Check sheet for the drawn part. Datum: minimum x, y, z corner. Units: mm. A direction names the side the tool comes from. Coordinates: 2 decimals unless noted, no trailing zeros. Loops run counter-clockwise (first coordinate to the right, second up) from the corner with the lowest first, then second, coordinate; pieces in that order, holes last.
Q1. Sectioned sample at D-D (x = 23.5). Enter the section's corners in (y, z).
Q2. Mould release check, pull along Z, two halves, no side actions. Record for the marked faces 1, 2 and 3: +Z half, -Z half, draft (parallel to the pull), parting line (faces both ways), or undercut.
Q3. Sectioned sample at C-C (z = 13.25). Enter the section's corners in (x, y), then the cut area to 3 significant figures.
Q4. Sectioned sample at B-B (y = 2.25). Count the separate pieces of the cut face and the enclosed holes in it, then the cut area to 3 significant figures.
Q5. Material ranges on probe 1 along X at (y, z) = (2.9, 13.25); probe 2 along X at (y, z) = (8.5, 13.25); probe 3 along Z at (x, y) = (42, 2.05), recorded low to high.
Q6. Access from +Z, -Z, +X, -X, +Y, -Y to the whole of each face (thin tool, end or side, straight path). Record for the marked faces 4, 5 and 6.
Q7. Go/stop test with flat-tipped pins: P1, Ø1.2, axis at x = 41.5, y = 2.5, coming from the +Z side; P2, Ø5, axis at x = 23.5, z = 13.25, coming from the +Y side; P3, Ø3.5, axis at x = 42, z = 12, coming from the +Y side; P4, Ø1.2, axis at x = 5.5, y = 2, coming from the +Z side. Record where each tip stops, or that it passes through.
Q8. Sectioned sample at A-A (x = 5). Enter the section's corners in (y, z).
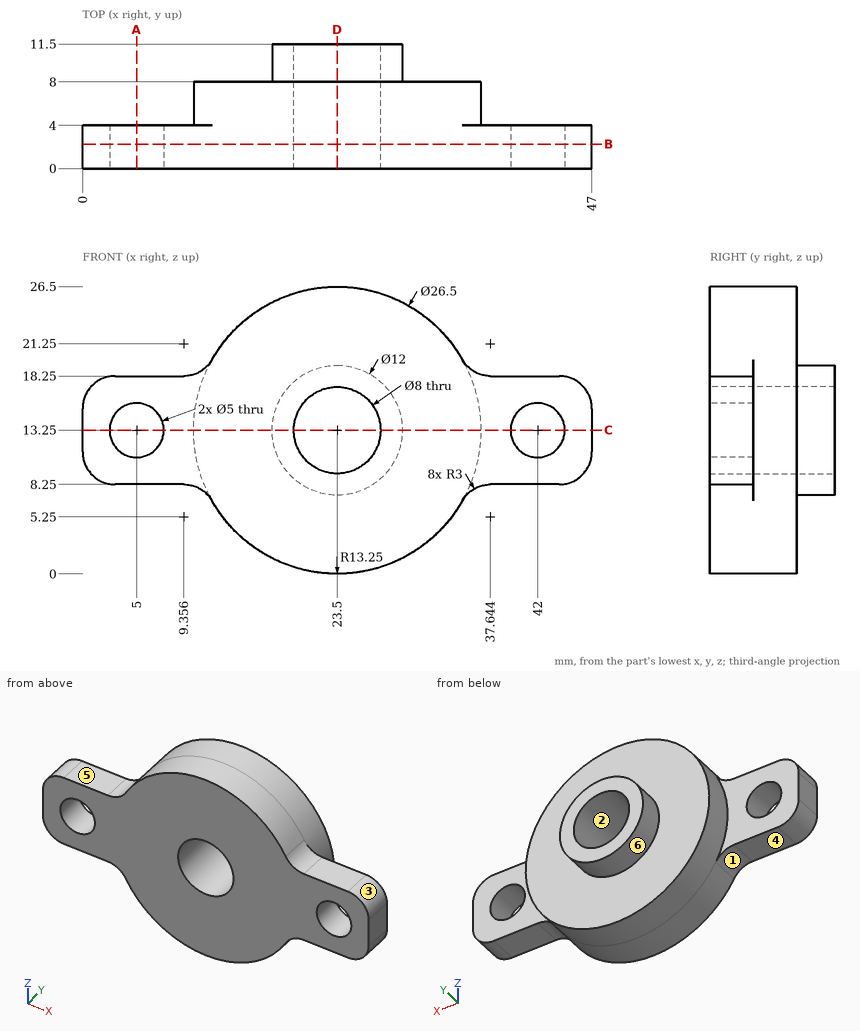
Geometry check:
1. outline: (0, 0) - (8, 0) - (8, 7.25) - (11.5, 7.25) - (11.5, 9.25) - (0, 9.25) - close; (0, 17.25) - (11.5, 17.25) - (11.5, 19.25) - (8, 19.25) - (8, 26.5) - (0, 26.5) - close
2. face 1: -Z half
2. face 2: undercut
2. face 3: +Z half
3. outline: (0, 0) - (2.5, 0) - (2.5, 4) - (0, 4) - close; (7.5, 0) - (19.5, 0) - (19.5, 11.5) - (17.5, 11.5) - (17.5, 8) - (10.25, 8) - (10.25, 4) - (7.5, 4) - close; (27.5, 0) - (39.5, 0) - (39.5, 4) - (36.75, 4) - (36.75, 8) - (29.5, 8) - (29.5, 11.5) - (27.5, 11.5) - close; (44.5, 0) - (47, 0) - (47, 4) - (44.5, 4) - close
3. area: 204 mm2
4. separate pieces: 1
4. enclosed holes: 3
4. area: 668 mm2
5. probe 1: x = 0 to 2.5, 7.5 to 19.5, 27.5 to 39.5, 44.5 to 47
5. probe 2: x = 17.5 to 19.5, 27.5 to 29.5
5. probe 3: z = 8.25 to 10.75, 15.75 to 18.25
6. face 4: -Z, -X, +Y, -Y
6. face 5: +Z, -X, +Y, -Y
6. face 6: +Y
7. P1: stops at z = 18.25
7. P2: passes through
7. P3: stops at y = 4
7. P4: stops at z = 18.25
8. outline: (0, 8.25) - (4, 8.25) - (4, 10.75) - (0, 10.75) - close; (0, 15.75) - (4, 15.75) - (4, 18.25) - (0, 18.25) - close
